Geometry check sheet. Reference: the model listing, model coordinates, mm. A direction names the side the tool comes from. Coordinates: 2 decimals unless noted, no trailing zeros. Loops run counter-clockwise (first coordinate to the right, second up) from the corner with the lowest first, then second, coordinate; pieces in that order, holes last. Notation, with made-up numbers: (37.5, 48.25) - (49.5, 48.25) arc R15 ccw to (49.5, 62.25) - close; hole circle Ø5 at (61, 56). An arc over 180 degrees is marked (long way). Write each question's results on one line, items separated by ' | '. Start each with the question number.
(1) Sectioned sample at A-A (y = -25). Enter the section's corners in (x, z), plus the area to 3 significant figures.
(2) Material ranges on probe 1 along Y at (x, z) = (0, 8.25); probe 2 along Z at (x, y) = (-20.5, -5); probe 3 along Y at (x, z) = (-3, 6.25), recorded low to high.
(3) Mould release check, pull along Z, two halves, no side actions. Record for faces 1 (the face through (-11.923, 3.755, 16.521)), 2 (the face through (-10, 8, 18)), 3 (the face through (-6.691, -12.864, 8.916)): pulls with the +Z half, pulls with the -Z half, needs draft (parallel to the pull), parting line crosses it, or undercut.
(4) Go/stop test with flat-tipped pins: pin 1 Ø6 at (x, z) = (-3, 10) entering from +Y; pin 2 Ø12 at (x, y) = (5.5, 11.5) entering from -Z; pin 3 Ø17.5 at (x, y) = (0, 0) entering from +Z; pin 4 Ø10 at (x, z) = (10, 14) entering from +Y. Record where each tip stops, or that it passes through.
(5) Sectioned sample at C-C (x = -11). Enter the section's corners in (y, z).
(6) Sectioned sample at D-D (y = -17). Enter the section's corners in (x, z).
(7) Sectioned sample at B-B (z = 9.25). Enter the section's corners in (x, y), plus the area to 3 significant figures.
(8) Access from +Z, -Z, +X, -X, +Y, -Y to the whole of each face (thin tool, end or side, straight path). Record for faces 4 (the face through (0, 0, 3)), 5 (the face through (0, 19, 3)), 6 (the face through (21.978, 11.863, 8.874)), 7 (the face through (-17, -10, 3)), 8 (the face through (15.48, -9.19, 8.92)).
from build123d import *

# Parameters (mm, degrees)
BASE_EXTRUDE_DEPTH           = 18
COMBUSTION_CHAMBER_PROFILE_R = 14.5
CUT_EXTRUDE1_DEPTH           = 12
SKETCH6_R                    = 12.5
CUT_EXTRUDE5_DEPTH           = 3


with BuildPart() as part:
    # rotor profile → Base-Extrude (new body)
    with BuildSketch(Plane.XY):
        with BuildLine():
            Line((-24.173095267, 13.130970823), (-22.181236737, 11.980970764))
            Line((-22.181236737, 11.980970764), (-21.823840171, 12.599999774))
            Line((-21.823840171, 12.599999774), (-21.466443413, 13.219029117))
            Line((-21.466443413, 13.219029117), (-23.458301944, 14.369029176))
            ThreePointArc((-23.458301944, 14.369029176), (-12.161921269, 19.163134144), (0, 20.8))
            ThreePointArc((0, 20.8), (12.161921269, 19.163134144), (23.458301944, 14.369029176))
            Line((23.458301944, 14.369029176), (19.128174925, 11.869029176))
            Line((19.128174925, 11.869029176), (19.485571586, 11.249999999))
            Line((19.485571586, 11.249999999), (19.842968249, 10.630970821))
            Line((19.842968249, 10.630970821), (24.173095268, 13.130970821))
            ThreePointArc((24.173095268, 13.130970821), (22.676721692, 0.95096574), (18.013328561, -10.399999953))
            ThreePointArc((18.013328561, -10.399999953), (10.514800547, -20.114099885), (0.714793524, -27.500000115))
            Line((0.714793524, -27.500000115), (0.714793524, -22.500000115))
            Line((0.714793524, -22.500000115), (0, -22.500000115))
            Line((0, -22.500000115), (-0.714793848, -22.500000115))
            Line((-0.714793848, -22.500000115), (-0.714793848, -27.500000115))
            ThreePointArc((-0.714793848, -27.500000115), (-10.514800813, -20.114099941), (-18.013328717, -10.400000004))
            ThreePointArc((-18.013328717, -10.400000004), (-22.676721717, 0.95096574), (-24.173095267, 13.130970823))
        make_face()
    extrude(amount=BASE_EXTRUDE_DEPTH)

    # combustion chamber profile → Cut-Extrude1 (cut)
    with BuildSketch(Plane(origin=(0, 0, 3), x_dir=(-1, 0, 0), z_dir=(0, 0, -1))):
        Circle(COMBUSTION_CHAMBER_PROFILE_R)
        Polygon((18, 21), (18, 18), (0, 18), (-18, 18), (-18, 21), align=None)
        Polygon((-9.186533479, -26.088457268), (-27.186533479, 5.088457268), (-24.588457268, 6.588457268), (-15.588457268, -9), (-6.588457268, -24.588457268), align=None)
        Polygon((27.186533479, 5.088457268), (9.186533479, -26.088457268), (6.588457268, -24.588457268), (15.588457268, -9), (24.588457268, 6.588457268), align=None)
    extrude(amount=-CUT_EXTRUDE1_DEPTH, mode=Mode.SUBTRACT)

    # Sketch6 → Cut-Extrude5 (cut)
    with BuildSketch(Plane(origin=(0, 0, 18), x_dir=(-1, 0, 0), z_dir=(0, 0, -1))):
        Circle(SKETCH6_R)
    extrude(amount=CUT_EXTRUDE5_DEPTH, mode=Mode.SUBTRACT)


solid = part.part
Outcome:
1) outline: (-4.68, 0) - (-0.71, 0) - (-0.71, 18) - (-4.68, 18) - close; (0.71, 0) - (4.68, 0) - (4.68, 18) - (0.71, 18) - close | area: 143 mm2
2) probe 1: y = -22.5 to -14.5, 14.5 to 18 | probe 2: z = 0 to 3, 15 to 18 | probe 3: y = -26.13 to -14.19, 14.19 to 18
3) face 1: needs draft | face 2: pulls with the +Z half | face 3: undercut
4) pin 1: stops at y = 18 | pin 2: stops at z = 0 | pin 3: stops at z = 3 | pin 4: stops at y = 20.52
5) outline: (-19.63, 0) - (19.47, 0) - (19.47, 3) - (18, 3) - (18, 15) - (19.47, 15) - (19.47, 18) - (5.94, 18) - (5.94, 15) - (9.45, 15) - (9.45, 3) - (-9.45, 3) - (-9.45, 15) - (-5.94, 15) - (-5.94, 18) - (-19.63, 18) - (-19.63, 15) - (-16.95, 15) - (-16.95, 3) - (-19.63, 3) - close
6) outline: (-13.39, 0) - (13.39, 0) - (13.39, 3) - (10.97, 3) - (10.97, 15) - (13.39, 15) - (13.39, 18) - (-13.39, 18) - (-13.39, 15) - (-10.97, 15) - (-10.97, 3) - (-13.39, 3) - close
7) outline: (-24.17, 13.13) arc R46 ccw to (-23.49, 4.69) - (-7.69, -22.69) arc R46 ccw to (-0.71, -27.5) - (-0.71, -22.5) - (0.71, -22.5) - (0.71, -27.5) arc R46 ccw to (7.69, -22.69) - (23.49, 4.69) arc R46 ccw to (24.17, 13.13) - (19.84, 10.63) - (19.13, 11.87) - (23.46, 14.37) arc R46 ccw to (15.8, 18) - (-15.8, 18) arc R46 ccw to (-23.46, 14.37) - (-21.47, 13.22) - (-22.18, 11.98) - close; hole circle Ø29 at (0, 0) | area: 826 mm2
8) face 4: none | face 5: +X, -X, +Y | face 6: +Z, -Z | face 7: -X, -Y | face 8: +X, -Y
